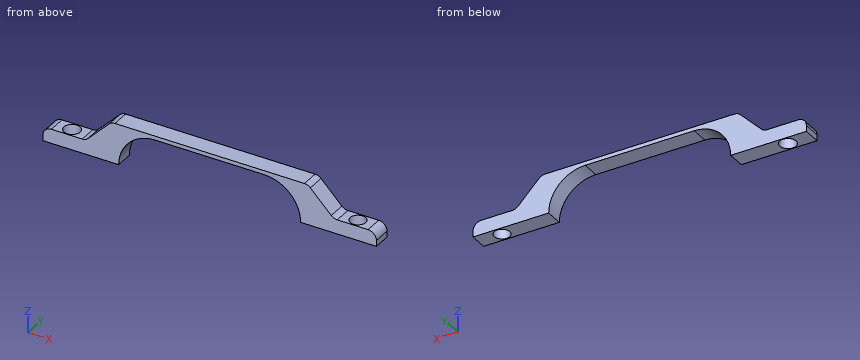
from build123d import *

# Parameters (mm, degrees)
F1_DEPTH = 2.7
F2_R     = 1.27
F3_R     = 1.25
F5_DEPTH = 2.165684
F4_R     = 1.2
F6_DEPTH = 2.165684


with BuildPart() as f1:
    # F0 (on Front) → F1 (new body)
    with BuildSketch(Plane.XZ):
        with BuildLine():
            Line((0, 2.164684), (0, 0))
            Line((0, 0), (11.5316, 0))
            ThreePointArc((11.5316, 0), (13.160848, 3.933352), (17.0942, 5.5626))
            Line((17.0942, 5.5626), (33.7058, 5.5626))
            ThreePointArc((33.7058, 5.5626), (37.639152, 3.933352), (39.2684, 0))
            Line((39.2684, 0), (50.8, 0))
            Line((50.8, 0), (50.8, 2.164684))
            Line((50.8, 2.164684), (44.297848, 2.164684))
            Line((44.297848, 2.164684), (40.37185, 6.1626))
            Line((40.37185, 6.1626), (10.42815, 6.1626))
            Line((10.42815, 6.1626), (6.502152, 2.164684))
            Line((6.502152, 2.164684), (0, 2.164684))
        make_face()
    extrude(amount=F1_DEPTH)

    # F2
    f2_edges = [f1.edges().sort_by_distance(p)[0] for p in [
        (50.8, -1.35, 2.164684),
        (44.297848, -1.35, 2.164684),
        (40.37185, -1.35, 6.1626),
        (10.42815, -1.35, 6.1626),
        (6.502152, -1.35, 2.164684),
        (0, -1.35, 2.164684),
    ]]
    fillet(f2_edges, radius=F2_R)

    # F3 (on face) → F5 (cut, through all)
    with BuildSketch(Plane.XY.offset(2.164684)):
        with Locations((3.619668, -1.35)):
            Circle(F3_R)
    extrude(amount=-F5_DEPTH, mode=Mode.SUBTRACT)

    # F4 (on face) → F6 (cut, through all)
    with BuildSketch(Plane.XY.offset(2.164684)):
        with Locations((47.180332, -1.35)):
            Circle(F4_R)
    extrude(amount=-F6_DEPTH, mode=Mode.SUBTRACT)


solid = f1.part
Design review of the part built by this model. Coordinates are the model's own, in mm. Give positions to 0.01 mm unless a question says otherwise; leave off trailing zeros. Order: outer loops, then holes, each group sorted by start corner. A loop starts at its lowest first (then second) coordinate and runs counter-clockwise, first axis right, second up. Notation, with made-up numbers: (74, -36.75) - (128, -36.75) arc R18 cw to (128, -6.75) - close; hole circle Ø1 at (3.25, 22.25). An arc over 180 degrees is marked (long way). Write item = value, one per line. Start each with the question number.
Q1. We need section C-C on x = 22.5. State the section outline as (y, z) points, plus the area to 3 significant figures.
Q2. To check wall thickness, follow L1, parallel to X at y = -2.15, z = 1; L2, parallel to X at y = -0.95, z = 2; L3, parallel to Z at x = 3, y = -0.2. State the ranges of each line that lie inside material, in increasing order. Write a range as from..to.
Q3. We need section A-A on y = -1.35. State the section outline as (x, z) points.
Q4. Clearance check with flat-ended pins moving along their axes: pin 1 Ø1 at (y, z) = (-2, 3.5) entering from +X; pin 2 Ø1.4 at (x, y) = (48, -0.5) entering from +Z. State where each tip first meets the part, or that it passes through.
Q5. We need section D-D on x = 43. State the section outline as (y, z) points.
Q6. We need section B-B on z = 1.5. State the section outline as (x, y) points, plus the area to 3 significant figures.
Working result:
q1.outline = (-2.7, 5.56) - (0, 5.56) - (0, 6.16) - (-2.7, 6.16) - close
q1.area = 1.62 mm²
q2.L1 = 0..2.66, 4.58..11.62, 39.18..46.29, 48.07..50.8
q2.L2 = 0.64..2.44, 4.8..11.9, 38.9..46.05, 48.31..50.16
q2.L3 = 0..2.16
q3.outline = (0, 0) - (2.37, 0) - (2.37, 2.16) - (1.27, 2.16) arc R1.27 ccw to (0, 0.89) - close; (4.87, 0) - (11.53, 0) arc R5.56 cw to (17.09, 5.56) - (33.71, 5.56) arc R5.56 cw to (39.27, 0) - (45.98, 0) - (45.98, 2.16) - (44.83, 2.16) arc R1.27 cw to (43.92, 2.54) - (40.75, 5.78) arc R1.27 ccw to (39.84, 6.16) - (10.96, 6.16) arc R1.27 ccw to (10.05, 5.78) - (6.88, 2.54) arc R1.27 cw to (5.97, 2.16) - (4.87, 2.16) - close; (48.38, 0) - (50.8, 0) - (50.8, 0.89) arc R1.27 ccw to (49.53, 2.16) - (48.38, 2.16) - close
q4.pin_1 = 43.48
q4.pin_2 = 2.16
q5.outline = (-2.7, 0) - (0, 0) - (0, 3.49) - (-2.7, 3.49) - close
q6.outline = (0.15, -2.7) - (11.74, -2.7) - (11.74, 0) - (0.15, 0) - close; (39.06, -2.7) - (50.65, -2.7) - (50.65, 0) - (39.06, 0) - close; hole circle Ø2.5 at (3.62, -1.35); hole circle Ø2.4 at (47.18, -1.35)
q6.area = 53.1 mm²
